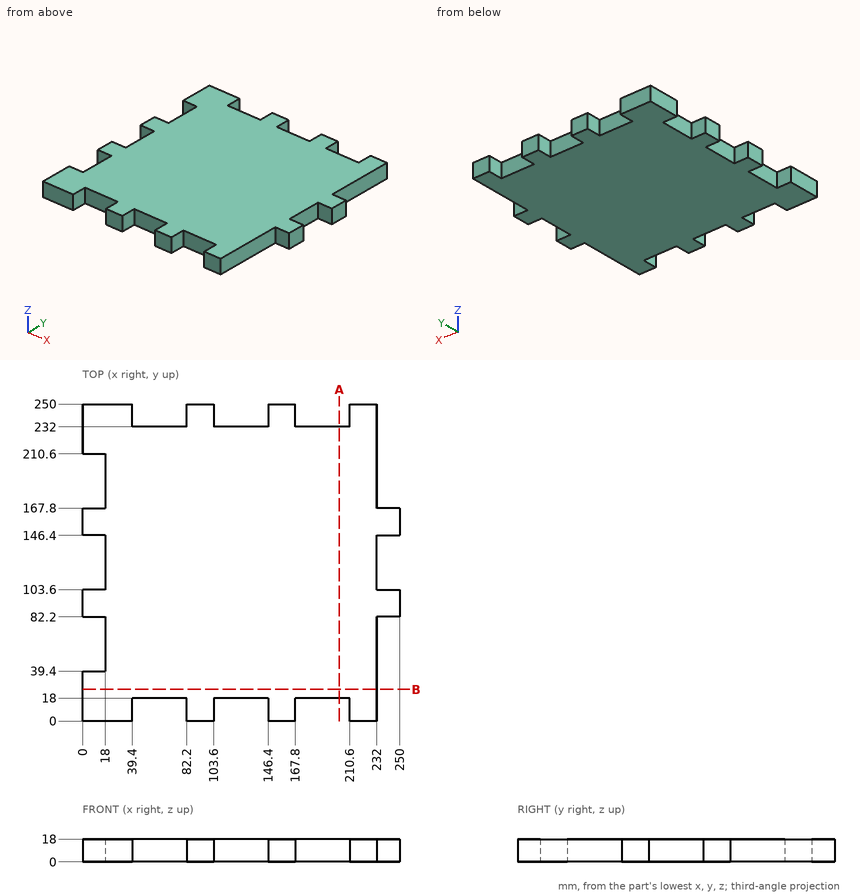
The figure shows three views and two pictorial views of one solid part (mm, origin at its lowest corner). Answer the questions. Round coordinates to 2 decimals unless told otherwise and drop trailing zeros. Write each loop counter-clockwise with the first axis right and the second up, starting at its lowest first coordinate (ties: lowest second). Pieces come first, ordered by that corner, then holes. Notation, with made-up numbers: (-11.75, -36) - (-4.75, -36) arc R17 ccw to (-4.75, -9) - close; hole circle Ø8 at (28, 12). An arc over 180 degrees is marked (long way). Use one line per item in the form item = value. Start each with the question number.
Item 1: Find the intervals of material crossed by line 1 (Y direction, x = 12, z = 9.25); line 2 (X direction, y = 237, z = 15); line 3 (X direction, y = 169, z = 5.5), in increasing order. Write a range as [from, to].
Item 2: A cutting plane is placed at A-A (x = 202.5). Write down the section's boundary in (y, z).
Item 3: A cutting plane is placed at B-B (y = 25). Write down the section's boundary in (x, z), plus the area to 3 significant figures.
Item 4: Flat-ended cylindrical pins translate along their axes: pin 1 Ø10 at (x, z) = (205, 13) entering from +Y; pin 2 Ø4 at (y, z) = (213.5, 2.5) entering from -X; pin 3 Ø9 at (y, z) = (11, 12.5) entering from +X; pin 4 Ø5.5 at (x, z) = (236.5, 12.5) entering from +Y. Find the tip coordinate at first contact, or state that the pin passes through.
The answers:
q1.line_1 = [0, 39.4], [82.2, 103.6], [146.4, 167.8], [210.6, 250]
q1.line_2 = [0, 39.4], [82.2, 103.6], [146.4, 167.8], [210.6, 232]
q1.line_3 = [18, 232]
q2.outline = (18, 0) - (232, 0) - (232, 18) - (18, 18) - close
q3.outline = (0, 0) - (232, 0) - (232, 18) - (0, 18) - close
q3.area = 4,180 mm^2
q4.pin_1 = 232
q4.pin_2 = 0
q4.pin_3 = 232
q4.pin_4 = 167.8
